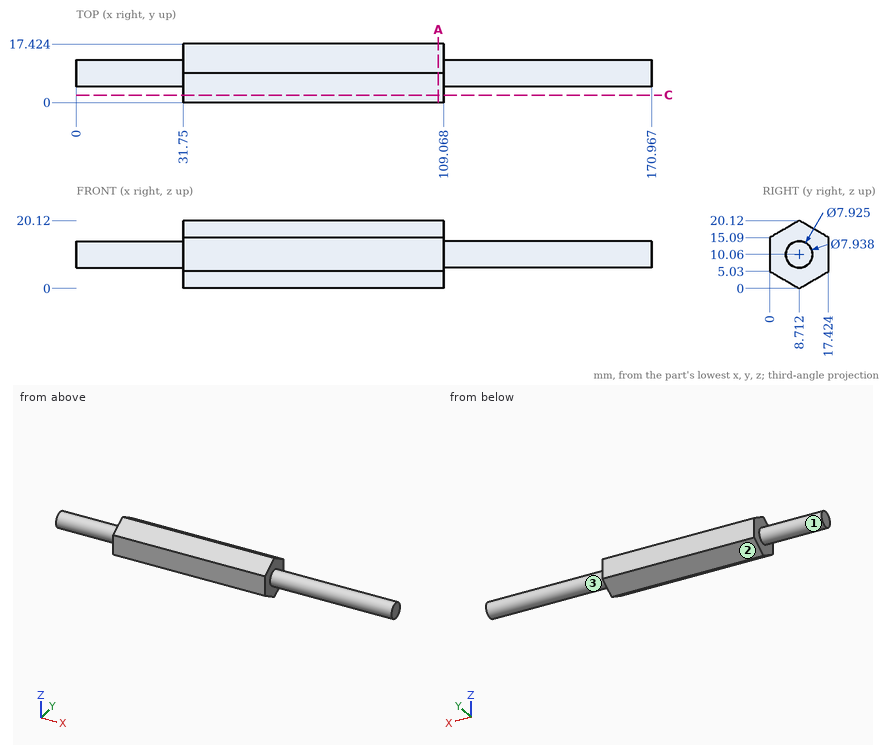
The drawing under review shows one solid part. Ordinate dimensions are in mm from its lowest x, y, z. A direction names the side the tool comes from. Give positions to 0.01 mm unless a question says otherwise; leave off trailing zeros. Write each loop counter-clockwise with the first axis right and the second up, starting at its lowest first coordinate (ties: lowest second). Pieces come first, ordered by that corner, then holes. Notation, with made-up numbers: M 46.25,-29 L 101.25,-29 A24 ccw 101.25,-11 Z; hole C -9.5,-18.75 d4. An arc over 180 degrees is marked long. Write each question's results on one line, items separated by ' | '. Start each with the question number.
1. Insertion check: pin 1 Ø8.5 at (y, z) = (5.5, 14) entering from -X; pin 2 Ø1.5 at (x, z) = (118.5, 16) entering from -Y; pin 3 Ø4 at (y, z) = (2.5, 16.5) entering from +X; pin 4 Ø6 at (x, y) = (130.5, 6.5) entering from -Z. Each pin has a flat end and moves straight along its axis. Give the tip position at first contact, or say it passes through.
2. For probe 1 along Y at (x, z) = (122, 9.5); probe 2 along X at (y, z) = (12.5, 17); probe 3 along Y at (x, z) = (131, 10.5), list the stretches that pass through material, from the lowest coordinate up. Write a range as [from, to].
3. For the marked faces 1, 2 and 3, list the 3-axis set-ups (+Z, -Z, +X, -X, +Y, -Y) from which the entire face can be reached by the end or side of a thin tool; tool diameter is ignored.
4. We need section A-A (x = 107.5). Write out the cut boundary in (y, z) (1 decimal).
5. We need section C-C (y = 2.25). Write out the cut boundary in (x, z).
Results found:
1) pin 1: stops at x = 0 | pin 2: passes through | pin 3: stops at x = 109.07 | pin 4: stops at z = 6.09
2) probe 1: y = [4.78, 12.64] | probe 2: x = [31.75, 109.07] | probe 3: y = [4.77, 12.66]
3) face 1: -X | face 2: -Z, +X, -X, +Y | face 3: +X
4) outline: M 0,5 L 8.7,0 L 17.4,5 L 17.4,15.1 L 8.7,20.1 L 0,15.1 Z
5) outline: M 31.75,3.73 L 109.07,3.73 L 109.07,16.39 L 31.75,16.39 Z
